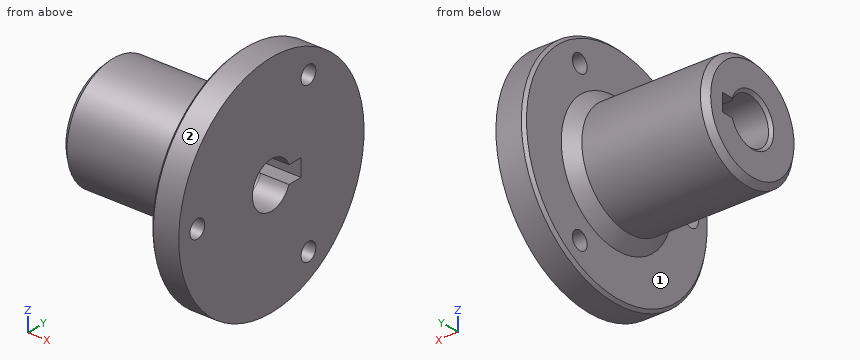
```python
from build123d import *

# Parameters (mm, degrees)
SKETCH_1_R          = 10
EXTRUDE_1_DEPTH     = 24
SKETCH_2_R          = 20
SKETCH_2_R_2        = 1.6
EXTRUDE_2_DEPTH     = 5
CHAMFER_1_SIZE      = 0.5
CHAMFER_2_SIZE      = 1
CHAMFER_3_SIZE      = 0.5
CHAMFER_4_SIZE      = 2
CUT_EXTRUDE_1_DEPTH = 10


with BuildPart() as part:
    # 草图1 → 凸台-拉伸1 (new body)
    with BuildSketch(Plane(origin=(0, 0, 0), x_dir=(0, 0, -1), z_dir=(1, 0, 0))):
        Circle(SKETCH_1_R)
        with BuildLine():
            Line((0, 6.4), (-1.55, 6.4))
            Line((-1.55, 6.4), (-1.55, 3.795721275))
            ThreePointArc((-1.55, 3.795721275), (0, -4.1), (1.55, 3.795721275))
            Line((1.55, 3.795721275), (1.55, 6.4))
            Line((1.55, 6.4), (0, 6.4))
        make_face(mode=Mode.SUBTRACT)
    extrude(amount=EXTRUDE_1_DEPTH)

    # 草图2 → 凸台-拉伸2 (add)
    with BuildSketch(Plane(origin=(24, 0, 0), x_dir=(0, 0, -1), z_dir=(1, 0, 0))):
        Circle(SKETCH_2_R)
        with Locations((-13.856406461, 8)):
            Circle(SKETCH_2_R_2, mode=Mode.SUBTRACT)
        with Locations((13.856406461, 8)):
            Circle(SKETCH_2_R_2, mode=Mode.SUBTRACT)
        with Locations((0, -16)):
            Circle(SKETCH_2_R_2, mode=Mode.SUBTRACT)
    extrude(amount=EXTRUDE_2_DEPTH)

    # 倒角1
    chamfer_1_edges = [part.edges().sort_by_distance(p)[0] for p in [
        (0, -4.1, 0),
    ]]
    chamfer(chamfer_1_edges, length=CHAMFER_1_SIZE)

    # 倒角2
    chamfer_2_edges = [part.edges().sort_by_distance(p)[0] for p in [
        (0, 0, 10),
    ]]
    chamfer(chamfer_2_edges, length=CHAMFER_2_SIZE)

    # 倒角3
    chamfer_3_edges = [part.edges().sort_by_distance(p)[0] for p in [
        (24, 0, 20),
    ]]
    chamfer(chamfer_3_edges, length=CHAMFER_3_SIZE)

    # 倒角4
    chamfer_4_edges = [part.edges().sort_by_distance(p)[0] for p in [
        (24, 0, 10),
    ]]
    chamfer(chamfer_4_edges, length=CHAMFER_4_SIZE)

    # 草图3 → 切除-拉伸1 (cut)
    with BuildSketch(Plane.ZY.offset(-24)):
        with BuildLine():
            Line((0, 6.4), (-1.55, 6.4))
            Line((-1.55, 6.4), (-1.55, 3.795721275))
            ThreePointArc((-1.55, 3.795721275), (0, -4.1), (1.55, 3.795721275))
            Line((1.55, 3.795721275), (1.55, 6.4))
            Line((1.55, 6.4), (0, 6.4))
        make_face()
    extrude(amount=-CUT_EXTRUDE_1_DEPTH, mode=Mode.SUBTRACT)


solid = part.part
```
Design review of the part built by this model. Coordinates are the model's own, in mm. Face numbers are marked on the shaded views. A direction names the side the tool comes from. Round coordinates to 2 decimals unless told otherwise and drop trailing zeros. Write each loop counter-clockwise with the first axis right and the second up, starting at its lowest first coordinate (ties: lowest second). Pieces come first, ordered by that corner, then holes.
Item 1: For the marked faces 1 and 2, list the 3-axis set-ups (+Z, -Z, +X, -X, +Y, -Y) from which the entire face can be reached by the end or side of a thin tool; tool diameter is ignored.
Item 2: For probe 1 along Y at (x, z) = (25.25, 0); probe 2 along X at (y, z) = (9, -11); probe 3 along Z at (x, y) = (9.5, -7), list the stretches that pass through material, from the lowest coordinate up.
Item 3: We need section B-B on x = 9.25. Write out the cut boundary in (y, z).
Item 4: We need section C-C on y = 8. State how many separate pieces and enclosed holes the cut face has, and give its area (3 significant figures).
Item 5: Clearance check with flat-ended pins moving along their axes: pin 1 Ø1.3 at (x, y) = (12.5, 5) entering from -Z; pin 2 Ø3 at (x, z) = (11, -3) entering from +Y; pin 3 Ø1.3 at (x, y) = (18.5, 5.5) entering from +Z. State where each tip first meets the part, or that it passes through.
Item 6: We need section A-A on z = 0. Write out the cut boundary in (x, y).
Returned:
1. face 1: -X
1. face 2: +X, -X
2. probe 1: y = -20 to -17.6, -14.4 to -4.1, 6.4 to 20
2. probe 2: x = 24 to 29
2. probe 3: z = -7.14 to 7.14
3. outline: circle Ø20 at (0, 0); hole (3.8, -1.55) - (6.4, -1.55) - (6.4, 1.55) - (3.8, 1.55) arc R4.1 ccw (long way) to start
4. separate pieces: 3
4. enclosed holes: 0
4. area: 443 mm2
5. pin 1: stops at z = -9
5. pin 2: stops at y = 9.89
5. pin 3: stops at z = 8.75
6. outline: (0, -9) - (1, -10) - (22, -10) - (24, -12) - (24, -14.4) - (29, -14.4) - (29, -4.1) - (0.5, -4.1) - (0, -4.6) - close; (0, 6.4) - (29, 6.4) - (29, 20) - (24.5, 20) - (24, 19.5) - (24, 12) - (22, 10) - (1, 10) - (0, 9) - close; (24, -19.5) - (24.5, -20) - (29, -20) - (29, -17.6) - (24, -17.6) - close
